Input: part model. Units: mm. Frame: model coordinates. Coordinates: 2 decimals unless noted, no trailing zeros. Loops run counter-clockwise (first coordinate to the right, second up) from the corner with the lowest first, then second, coordinate; pieces in that order, holes last.
Autodesk Inventor part; units mm, degrees
ref_plane "YZ Plane" through (0, 0, 0) normal (1, 0, 0) x (0, 1, 0)
ref_plane "XZ Plane" through (0, 0, 0) normal (0, 1, 0) x (-1, 0, 0)
ref_plane "XY Plane" through (0, 0, 0) normal (0, 0, 1) x (1, 0, 0)
sketch "Sketch1" plane through (0, 0, 0) normal (0, 0, 1) x (1, 0, 0)
  line L0 (0, 0) -> (24, 0)
  circle A0 centre (0, 0) radius 1.6
  line L1 (0, 0) -> (24, 0) construction
  line L2 (0, -3) -> (24, -3)
  line L3 (24, 3) -> (0, 3)
  arc A1 (0, 3) -> (0, -3) centre (0, 0) ccw
  line L4 (24, 0) -> (28, 0)
  circle A2 centre (27, 0) radius 1.6
  line L5 (27, 0) -> (0, 0) construction
  line L6 (27, 3) -> (0, 3)
  line L7 (0, -3) -> (27, -3)
  arc A3 (27, -3) -> (27, 3) centre (27, 0) ccw
  arc A4 (0, 3) -> (0, -3) centre (0, 0) ccw
  point P0 (12, 0)
  point P1 (13.5, 0)
  dimension "d0" = 24
  dimension "d1" = 3.2
  dimension "d6" = 4
  dimension "d7" = 3.2
  dimension "d8" = 6
extrude "Extrusion1" [suppressed]
sketch "Sketch2" plane through (0, 0, 0) normal (0, 0, 1) x (1, 0, 0)
  line L0 (0, 0) -> (28, 0)
  circle A0 centre (0, 0) radius 1.65
  circle A1 centre (28, 0) radius 1.65
  line L1 (0, 0) -> (28, 0) construction
  line L2 (0, -3) -> (28, -3)
  line L3 (28, 3) -> (0, 3)
  arc A2 (0, 3) -> (0, -3) centre (0, 0) ccw
  arc A3 (28, -3) -> (28, 3) centre (28, 0) ccw
  point P0 (14, 0)
  dimension "d9" = 28
  dimension "d10" = 3.3
  dimension "d11" = 3.3
  dimension "d12" = 6
extrude "Extrusion2" add sketch "Sketch2" along normal blind 3
sketch "Sketch3" plane through (0, 0, 3) normal (0, 0, 1) x (1, 0, 0)
  circle A0 centre (28, 0) radius 1.65
  line L0 (28, 0) -> (43, 0)
  line L1 (28, 0) -> (43, 0) construction
  line L2 (28, -3) -> (43, -3)
  line L3 (43, 3) -> (28, 3)
  arc A1 (28, 3) -> (28, -3) centre (28, 0) ccw
  arc A2 (43, -3) -> (43, 3) centre (43, 0) ccw
  circle A3 centre (43, 0) radius 1.65
  point P0 (0, 0)
  point P1 (35.5, 0)
  dimension "d15" = 15
  dimension "d16" = 6
extrude "Extrusion3" add sketch "Sketch3" against normal blind 3 contours A0 | A1 L3 A2 L2
sketch "Sketch4" plane through (0, 0, 3) normal (0, 0, 1) x (1, 0, 0)
  line L0 (38.0198, 0) -> (46.7499, 0)
  circle A0 centre (46.7499, 0) radius 1.65
  line L1 (0, 0) -> (46.7499, 0) construction
  line L2 (0, -3) -> (46.7499, -3)
  line L3 (46.7499, 3) -> (0, 3)
  arc A1 (0, 3) -> (0, -3) centre (0, 0) ccw
  arc A2 (46.7499, -3) -> (46.7499, 3) centre (46.7499, 0) ccw
  line L4 (39.9731, -3) -> (39.9731, 3)
  point P0 (23.375, 0)
  dimension "d19" = 3.3
  dimension "d20" = 6
extrude "Extrusion4" add sketch "Sketch4" against normal blind 3 contours L4 L3 A2 L2
extrude "Extrusion5" cut sketch "Sketch4" against normal blind 3 contours A0
sketch "Sketch5" plane through (0, 0, 3) normal (0, 0, 1) x (1, 0, 0)
  arc A0 (46.7499, -3) -> (46.7499, 3) centre (46.7499, 0) ccw
  line L0 (46.7499, 0) -> (54.7499, 0)
  circle A1 centre (54.7499, 0) radius 1.65
  line L1 (33.9937, 0) -> (54.7499, 0) construction
  line L2 (33.9937, 3) -> (54.7499, 3)
  line L3 (54.7499, -3) -> (33.9937, -3)
  arc A2 (33.9937, 3) -> (33.9937, -3) centre (33.9937, 0) ccw
  arc A3 (54.7499, -3) -> (54.7499, 3) centre (54.7499, 0) ccw
  point P0 (0, 0)
  point P1 (44.3718, 0)
  dimension "d25" = 8
  dimension "d26" = 3.3
extrude "Extrusion6" add sketch "Sketch5" against normal blind 3
properties part number "connector"
Item 1: Section query B-B (z = 0.8). Output: boundary loops of the cut face in (x, y).
Result:
outline: (0, -3) - (54.75, -3) arc R3 ccw to (54.75, 3) - (0, 3) arc R3 ccw to start; hole circle Ø3.3 at (0, 0); hole circle Ø3.3 at (54.75, 0)
Item 2: Section query C-C (y = 2.4). Output: boundary loops of the cut face in (x, z), then the cut area to 3 significant figures.
Result:
outline: (-1.8, 0) - (56.55, 0) - (56.55, 3) - (-1.8, 3) - close
area: 175 mm2
Item 3: Line query: L1, parallel to X at y = -0.2, z = 2.1; L2, parallel to Y at x = 0, z = 2.3; L3, parallel to X at y = 0.6, z = 2.1. Output: solid intervals per line, ascending.
Result:
L1: x = -2.99 to -1.64, 1.64 to 53.11, 56.39 to 57.74
L2: y = -3 to -1.65, 1.65 to 3
L3: x = -2.94 to -1.54, 1.54 to 53.21, 56.29 to 57.69
Item 4: Mould query, pull axis X, two halves, no side actions, for faces 1 (the face through (28, 3, 1)), 2 (the face through (57.75, -0.07, 1.52)), 3 (the face through (-1.216, -1.115, 1.479)). Classes: +X half, -X half, draft (parallel to the pull), parting line (faces both ways), or undercut.
Result:
face 1: draft
face 2: +X half
face 3: undercut
Item 5: Section query A-A (y = 0). Output: boundary loops of the cut face in (x, z), then the cut area to 3 significant figures.
Result:
outline: (-3, 0) - (-1.65, 0) - (-1.65, 3) - (-3, 3) - close; (1.65, 0) - (53.1, 0) - (53.1, 3) - (1.65, 3) - close; (56.4, 0) - (57.75, 0) - (57.75, 3) - (56.4, 3) - close
area: 162 mm2
